CAD build for the part. Positions are in the model's coordinates, mm. Round coordinates to 2 decimals unless told otherwise and drop trailing zeros. Write each loop counter-clockwise with the first axis right and the second up, starting at its lowest first coordinate (ties: lowest second). Pieces come first, ordered by that corner, then holes. Notation, with made-up numbers: (-19.5, 10) - (18.5, 10) arc R28 ccw to (18.5, 42) - close; hole circle Ø9 at (35, -25). An arc over 180 degrees is marked (long way). Use one line per item in the form item = value. Start each with the question number.
Item 1: Band-saw the part on A-A, the plane z = 11.5. List the corners of the cut face in (x, y), and give its area (3 significant figures).
Item 2: Drill centre lines: L1, parallel to Y at x = 0, z = 7.5; L2, parallel to X at y = -5.5, z = 2.25; L3, parallel to Y at x = 7, z = 9. Where is each one in solid material? Low to high.
Item 3: Pin check, flat tips, straight feed: pin 1 (2 mm diameter, centred on y = 10, z = 7, fed in from +X); pin 2 (8 mm diameter, centred on x = -0.5, y = 3.5, fed in from -Z); pin 3 (3 mm diameter, centred on y = -5.5, z = 1.5, fed in from -X). Stop position of each tip, or through.
Item 4: Pull direction X, two halves, no side cores. Call faces 1 (the conical face through (8.94, -15.58, 14.63)), 2 (the cylindrical face through (-2.17, -9.76, 7.4)), 3 (the conical face through (-8.94, -15.58, 0.37)): +X half, -X half, draft (parallel to the pull), parting line (faces both ways), or undercut.
from build123d import *

# Parameters (mm, degrees)
SKETCH2_R               = 10
BOSS_EXTRUDE1_DEPTH     = 15
SKETCH3_OUTSIDE_W       = 104.962
SKETCH3_OUTSIDE_H       = 99.604
SKETCH3_OUTSIDE_R       = 17.320508076
CUT_EXTRUDE1_DEPTH      = 15
CUT_EXTRUDE1_DRAFT      = -60
MIRROR1_COPY_1_SKETCH_W = 104.962
MIRROR1_COPY_1_SKETCH_H = 99.604
MIRROR1_COPY_1_SKETCH_R = 17.320508076
MIRROR1_COPY_1_DEPTH    = 15
MIRROR1_COPY_1_DRAFT    = -60


with BuildPart() as part:
    # Sketch2 → Boss-Extrude1 (new body)
    with BuildSketch(Plane.XY):
        Polygon((20, 0), (10, 17.320508076), (-10, 17.320508076), (-20, 0), (-10, -17.320508076), (10, -17.320508076), align=None)
        Circle(SKETCH2_R, mode=Mode.SUBTRACT)
    extrude(amount=BOSS_EXTRUDE1_DEPTH)


with BuildPart() as cut_extrude1_tool:
    # Sketch3 outside → Cut-Extrude1 (with draft: the straight prism first)
    with BuildSketch(Plane(origin=(0, 0, 0), x_dir=(-1, 0, 0), z_dir=(0, 0, -1))):
        Rectangle(SKETCH3_OUTSIDE_W, SKETCH3_OUTSIDE_H)
        Circle(SKETCH3_OUTSIDE_R, mode=Mode.SUBTRACT)
    extrude(amount=-CUT_EXTRUDE1_DEPTH)
    # Cut-Extrude1: the draft: its side faces are tilted about the plane it starts from
    cut_extrude1_sides = [cut_extrude1_tool.faces().sort_by_distance(p)[0] for p in [
        (0, -49.802, 7.5),
        (-52.481, 0, 7.5),
        (0, 49.802, 7.5),
        (52.481, 0, 7.5),
        (17.320508076, 0, 7.5),
    ]]
    draft(cut_extrude1_sides, Plane(origin=(0, 0, 0), x_dir=(-1, 0, 0), z_dir=(0, 0, -1)), CUT_EXTRUDE1_DRAFT)


with BuildPart() as part_1:
    add(part.part)

    # Cut-Extrude1: cut by cut_extrude1_tool
    add(cut_extrude1_tool.part, mode=Mode.SUBTRACT)


with BuildPart() as mirror1_copy_1_tool:
    # Mirror1 copy 1 sketch → Mirror1 copy 1 (with draft: the straight prism first)
    with BuildSketch(Plane(origin=(0, 0, 15), x_dir=(-1, 0, 0), z_dir=(0, 0, 1))):
        Rectangle(MIRROR1_COPY_1_SKETCH_W, MIRROR1_COPY_1_SKETCH_H)
        Circle(MIRROR1_COPY_1_SKETCH_R, mode=Mode.SUBTRACT)
    extrude(amount=-MIRROR1_COPY_1_DEPTH)
    # Mirror1 copy 1: the draft: its side faces are tilted about the plane it starts from
    mirror1_copy_1_sides = [mirror1_copy_1_tool.faces().sort_by_distance(p)[0] for p in [
        (0, -49.802, 7.5),
        (-52.481, 0, 7.5),
        (0, 49.802, 7.5),
        (52.481, 0, 7.5),
        (17.320508076, 0, 7.5),
    ]]
    draft(mirror1_copy_1_sides, Plane(origin=(0, 0, 15), x_dir=(-1, 0, 0), z_dir=(0, 0, 1)), MIRROR1_COPY_1_DRAFT)


with BuildPart() as part_2:
    add(part_1.part)

    # Mirror1 copy 1: cut by mirror1_copy_1_tool
    add(mirror1_copy_1_tool.part, mode=Mode.SUBTRACT)


solid = part_2.part
Determined:
q1.outline = (-20, 0) - (-10, -17.32) - (10, -17.32) - (20, 0) - (10, 17.32) - (-10, 17.32) - close; hole circle Ø20 at (0, 0)
q1.area = 725 mm²
q2.L1 = -17.32 to -10, 10 to 17.32
q2.L2 = -16.82 to -8.35, 8.35 to 16.82
q2.L3 = -17.32 to -7.14, 7.14 to 17.32
q3.pin_1 = 14.8
q3.pin_2 = through
q3.pin_3 = -17.69
q4.face_1 = +X half
q4.face_2 = undercut
q4.face_3 = -X half
